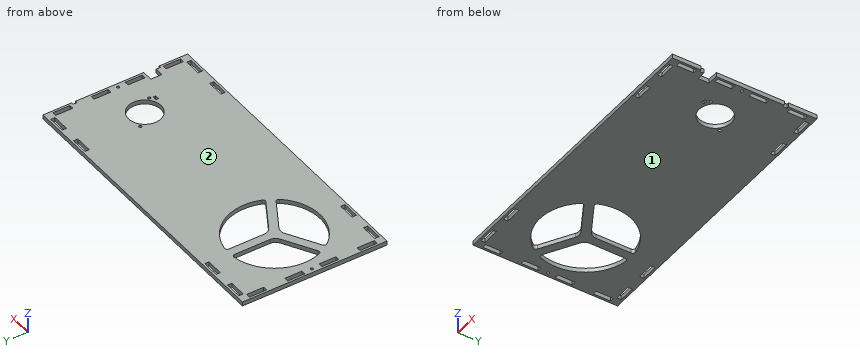
from build123d import *

# Parameters (mm, degrees)
F1_W     = 20
F1_H     = 5
F1_W_2   = 5
F1_H_2   = 20
F1_H_3   = 3
F1_R     = 1.6
F1_R_2   = 19
F2_DEPTH = 5


with BuildPart() as f2:
    # F1 (on Top) → F2 (new body)
    with BuildSketch(Plane.XY):
        Polygon((0, 170), (0, 0), (350, 0), (350, 33.5), (347.5, 33.5), (347.5, 38.5), (337.5, 38.5), (337.5, 51.5), (350, 51.5), (350, 131.5), (347.5, 131.5), (347.5, 136.5), (350, 136.5), (350, 170), align=None)
        with Locations((20, 5)):
            Rectangle(F1_W, F1_H, mode=Mode.SUBTRACT)
        with Locations((5, 20)):
            Rectangle(F1_W_2, F1_H_2, mode=Mode.SUBTRACT)
        with Locations((60, 5)):
            Rectangle(F1_W, F1_H, mode=Mode.SUBTRACT)
        with BuildLine():
            ThreePointArc((112.4804290917, 51.1232559442), (70.75, 31.25), (29.0195709083, 51.1232559442))
            ThreePointArc((29.0195709083, 51.1232559442), (28.3986145368, 53.5589638456), (29.8487111366, 55.6121271726))
            Line((29.8487111366, 55.6121271726), (65.75, 76.3397459622))
            ThreePointArc((65.75, 76.3397459622), (70.75, 77.6794919243), (75.75, 76.3397459622))
            Line((75.75, 76.3397459622), (111.6512888634, 55.6121271726))
            ThreePointArc((111.6512888634, 55.6121271726), (113.1013854632, 53.5589638456), (112.4804290917, 51.1232559442))
        make_face(mode=Mode.SUBTRACT)
        with Locations((5, 65)):
            Rectangle(F1_W_2, F1_H_2, mode=Mode.SUBTRACT)
        with Locations((290, 5)):
            Rectangle(F1_W, F1_H, mode=Mode.SUBTRACT)
        with Locations((330, 5)):
            Rectangle(F1_W, F1_H, mode=Mode.SUBTRACT)
        with Locations((345, 20)):
            Rectangle(F1_W_2, F1_H_2, mode=Mode.SUBTRACT)
        with Locations((310.775873661, 63.5)):
            Rectangle(F1_W_2, F1_H_3, mode=Mode.SUBTRACT)
        with Locations((314.25, 69)):
            Circle(F1_R, mode=Mode.SUBTRACT)
        with Locations((345, 65)):
            Rectangle(F1_W_2, F1_H_2, mode=Mode.SUBTRACT)
        with Locations((5, 85)):
            Circle(F1_R, mode=Mode.SUBTRACT)
        with Locations((5, 105)):
            Rectangle(F1_W_2, F1_H_2, mode=Mode.SUBTRACT)
        with BuildLine():
            Line((65.75, 135.1154916169), (65.75, 93.6602540378))
            ThreePointArc((65.75, 93.6602540378), (64.4102540378, 88.6602540378), (60.75, 85))
            Line((60.75, 85), (24.8487111366, 64.2723812105))
            ThreePointArc((24.8487111366, 64.2723812105), (22.3455712374, 64.0431423806), (20.5466645043, 65.7987603236))
            ThreePointArc((20.5466645043, 65.7987603236), (24.2011345466, 111.875), (62.2770935961, 138.0779837321))
            ThreePointArc((62.2770935961, 138.0779837321), (64.6969567006, 137.3978937738), (65.75, 135.1154916169))
        make_face(mode=Mode.SUBTRACT)
        with BuildLine():
            ThreePointArc((80.75, 85), (77.0897459622, 88.6602540378), (75.75, 93.6602540378))
            Line((75.75, 93.6602540378), (75.75, 135.1154916169))
            ThreePointArc((75.75, 135.1154916169), (76.8030432994, 137.3978937738), (79.2229064039, 138.0779837321))
            ThreePointArc((79.2229064039, 138.0779837321), (117.2988654534, 111.875), (120.9533354957, 65.7987603236))
            ThreePointArc((120.9533354957, 65.7987603236), (119.1544287626, 64.0431423806), (116.6512888634, 64.2723812105))
            Line((116.6512888634, 64.2723812105), (80.75, 85))
        make_face(mode=Mode.SUBTRACT)
        with Locations((5, 150)):
            Rectangle(F1_W_2, F1_H_2, mode=Mode.SUBTRACT)
        with Locations((20, 165)):
            Rectangle(F1_W, F1_H, mode=Mode.SUBTRACT)
        with Locations((60, 165)):
            Rectangle(F1_W, F1_H, mode=Mode.SUBTRACT)
        with Locations((298.25, 85)):
            Circle(F1_R_2, mode=Mode.SUBTRACT)
        with Locations((282.25, 101)):
            Circle(F1_R, mode=Mode.SUBTRACT)
        with Locations((345, 85)):
            Circle(F1_R, mode=Mode.SUBTRACT)
        with Locations((345, 105)):
            Rectangle(F1_W_2, F1_H_2, mode=Mode.SUBTRACT)
        with Locations((290, 165)):
            Rectangle(F1_W, F1_H, mode=Mode.SUBTRACT)
        with Locations((345, 150)):
            Rectangle(F1_W_2, F1_H_2, mode=Mode.SUBTRACT)
        with Locations((330, 165)):
            Rectangle(F1_W, F1_H, mode=Mode.SUBTRACT)
    extrude(amount=F2_DEPTH)


solid = f2.part
Could you check a few things on this model? Use its own coordinates, in mm. Face numbers are marked on the shaded views. Coordinates: 2 decimals unless noted, no trailing zeros. Order: outer loops, then holes, each group sorted by start corner. A loop starts at its lowest first (then second) coordinate and runs counter-clockwise, first axis right, second up. Notation, with made-up numbers: (24, 8) -> (77, 8) arc R36 ccw to (77, 44) -> close; hole circle Ø1 at (-16, -4.5). An arc over 180 degrees is marked (long way). One line per item, written item: value. Start each with the question number.
1) Imagine slicing it at B-B on z = 3.55. Count the separate pieces of the cut face and the enclosed holes in it, plus the area to 3 significant figures.
2) Imagine slicing it at A-A on y = 22. List the corners of the cut face in (x, z) for me, plus the area to 3 significant figures.
3) We'd pull the mould along Z, two halves only. Please class the marked faces 1 and 2: +Z half, -Z half, draft (parallel to the pull), parting line (faces both ways), or undercut.
4) If I drill on L1, parallel to Y at x = 16, z = 4.85; L2, parallel to X at y = 153, z = 4.25; L3, parallel to Y at x = 5, z = 3.8, over which ranges is the centre line in solid material (lowest first)? Write a range as [from, to].
5) I'm going to push a flat-ended pin straight in: pin 1 (2.5 mm diameter, centred on x = 345, y = 85, fed in from +Z) (3 decimals). Where does the tip first touch, or does it pass through?
Answer list:
1. separate pieces: 1
1. enclosed holes: 25
1. area: 49,100 mm2
2. outline: (0, 0) -> (2.5, 0) -> (2.5, 5) -> (0, 5) -> close; (7.5, 0) -> (342.5, 0) -> (342.5, 5) -> (7.5, 5) -> close; (347.5, 0) -> (350, 0) -> (350, 5) -> (347.5, 5) -> close
2. area: 1,700 mm2
3. face 1: -Z half
3. face 2: +Z half
4. L1: y = [0, 2.5], [7.5, 162.5], [167.5, 170]
4. L2: x = [0, 2.5], [7.5, 342.5], [347.5, 350]
4. L3: y = [0, 10], [30, 55], [75, 83.4], [86.6, 95], [115, 140], [160, 170]
5. pin 1: passes through
